Print and shaded views of the part. All mm, measured from the part's lowest x, y and z. Coordinates: 2 decimals unless noted, no trailing zeros. Loops run counter-clockwise (first coordinate to the right, second up) from the corner with the lowest first, then second, coordinate; pieces in that order, holes last. Notation, with made-up numbers: (3.5, -15.75) -> (47.5, -15.75) arc R5 ccw to (47.5, -9.75) -> close; hole circle Ø8 at (14.25, 17). An arc over 180 degrees is marked (long way). One line per question, with ' | ' between items. Start each with the question number.
1) Probe L1, parallel to X at y = 46.5, z = 0.7; L2, parallel to X at y = 37, z = 4; L3, parallel to Y at x = 240, z = 4.6. List the from-to ranges inside material, lowest first. Write a range as from..to.
2) Cut at C-C (z = 2.6). List the corners of the cut face in (x, y).
3) Cut at A-A (y = 47). List the corners of the cut face in (x, z).
4) Cut at D-D (x = 210.5). List the corners of the cut face in (y, z).
5) Drop flat-ended pins along their axis: pin 1 (2.5 mm diameter, centred on y = 36.5, z = 2, fed in from +X); pin 2 (3 mm diameter, centred on y = 47, z = 2, fed in from -X); pin 3 (3 mm diameter, centred on x = 259, z = 4, fed in from -Y). Give the stop position or say it passes through.
6) Cut at B-B (x = 237.5). List the corners of the cut face in (y, z), plus the area to 3 significant figures.
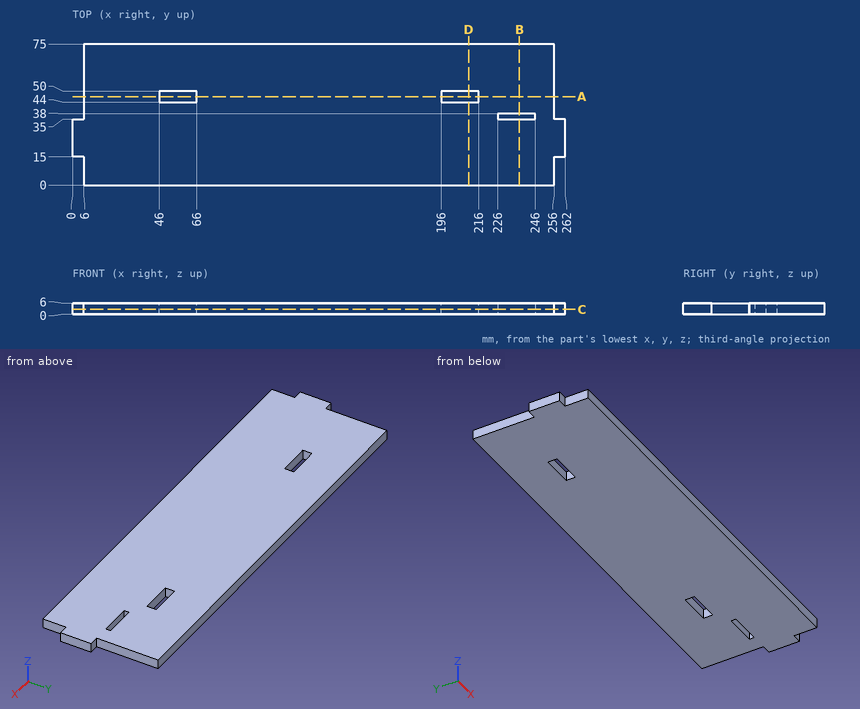
Reported:
1) L1: x = 6..46, 66..196, 216..256 | L2: x = 6..226, 246..256 | L3: y = 0..35, 38..75
2) outline: (0, 15) -> (6, 15) -> (6, 0) -> (256, 0) -> (256, 15) -> (262, 15) -> (262, 35) -> (256, 35) -> (256, 75) -> (6, 75) -> (6, 35) -> (0, 35) -> close; hole (46, 44) -> (66, 44) -> (66, 50) -> (46, 50) -> close; hole (196, 44) -> (216, 44) -> (216, 50) -> (196, 50) -> close; hole (226, 35) -> (246, 35) -> (246, 38) -> (226, 38) -> close
3) outline: (6, 0) -> (46, 0) -> (46, 6) -> (6, 6) -> close; (66, 0) -> (196, 0) -> (196, 6) -> (66, 6) -> close; (216, 0) -> (256, 0) -> (256, 6) -> (216, 6) -> close
4) outline: (0, 0) -> (44, 0) -> (44, 6) -> (0, 6) -> close; (50, 0) -> (75, 0) -> (75, 6) -> (50, 6) -> close
5) pin 1: stops at x = 256 | pin 2: stops at x = 6 | pin 3: stops at y = 15
6) outline: (0, 0) -> (35, 0) -> (35, 6) -> (0, 6) -> close; (38, 0) -> (75, 0) -> (75, 6) -> (38, 6) -> close | area: 432 mm²
